from build123d import *

# Parameters (mm, degrees)
F0_W           = 150
F0_H           = 35
F0_R           = 1.25
F0_R_2         = 0.9
F1_DEPTH       = 3
F2_R           = 5
F4_D           = 3.3
F4_CSINK_D     = 6.72
F4_CSINK_ANGLE = 90


with BuildPart() as f1:
    # F0 (on Top) → F1 (new body)
    with BuildSketch(Plane.XY):
        with Locations((75, 17.5)):
            Rectangle(F0_W, F0_H)
        with Locations((12, 15)):
            Circle(F0_R, mode=Mode.SUBTRACT)
        with Locations((45, 15)):
            Circle(F0_R, mode=Mode.SUBTRACT)
        with Locations((61, 15)):
            Circle(F0_R_2, mode=Mode.SUBTRACT)
        with Locations((101, 15)):
            Circle(F0_R_2, mode=Mode.SUBTRACT)
        with Locations((115, 23)):
            Circle(F0_R_2, mode=Mode.SUBTRACT)
    extrude(amount=F1_DEPTH)

    # F2
    f2_edges = [f1.edges().sort_by_distance(p)[0] for p in [
        (0, 35, 1.5),
        (0, 0, 1.5),
        (150, 0, 1.5),
        (150, 35, 1.5),
    ]]
    fillet(f2_edges, radius=F2_R)

    # F4 (through all)
    with Locations(Plane.XY.offset(3)):
        with Locations((5, 5), (145, 30)):
            CounterSinkHole(F4_D / 2, F4_CSINK_D / 2, counter_sink_angle=F4_CSINK_ANGLE)


solid = f1.part
The listing builds one solid part. Answer for the finished solid, in the listing's coordinates (mm). Coordinates: 2 decimals unless noted, no trailing zeros. Loops run counter-clockwise (first coordinate to the right, second up) from the corner with the lowest first, then second, coordinate; pieces in that order, holes last.
1) Find section A-A on x = 12. Write down the section's boundary in (y, z), then the cut area to 3 significant figures.
2) Determine the mould class of faces 1 (the face through (6.31, 4, 0.64)), 2 (the face through (148, 34, 2)), 3 (the face through (74, 0, 1)) for opening direction X: pulls with the +X half, pulls with the -X half, needs draft (parallel to the pull), parting line crosses it, or undercut.
3) A flat-ended cylindrical pin translates along its axis: pin 1 Ø1.1 at (x, y) = (115, 23) entering from +Z. Find the tip coordinate at first contact, or state that the pin passes through.
4) Find the intervals of material crossed by L1, parallel to Y at x = 12, z = 2.4; L2, parallel to Y at x = 61, z = 2.05; L3, parallel to X at y = 30, z = 0.9, in increasing order.
Values:
1. outline: (0, 0) - (13.75, 0) - (13.75, 3) - (0, 3) - close; (16.25, 0) - (35, 0) - (35, 3) - (16.25, 3) - close
1. area: 97.5 mm2
2. face 1: undercut
2. face 2: pulls with the +X half
2. face 3: needs draft
3. pin 1: passes through
4. L1: y = 0 to 13.75, 16.25 to 35
4. L2: y = 0 to 14.1, 15.9 to 35
4. L3: x = 0 to 143.35, 146.65 to 150
